```python
from build123d import *

# Parameters (mm, degrees)
ESBO_O1_R                = 2.5
RESSALTO_EXTRUS_O1_DEPTH = 1.26


with BuildPart() as part:
    # Esboço1 → Ressalto-extrusão1 (new body)
    with BuildSketch(Plane(origin=(0, 0, 0), x_dir=(1, 0, 0), z_dir=(0, 1, 0))):
        Polygon((-17.5, -9), (14.671572875, -9), (17.5, -7), (17.5, 9), (-17.5, 9), align=None)
        with Locations(Location((3.5, -1, 0), (0, 0, 270))):
            Circle(ESBO_O1_R, mode=Mode.SUBTRACT)
        with Locations(Location((-11.5, -1, 0), (0, 0, 270))):
            Circle(ESBO_O1_R, mode=Mode.SUBTRACT)
    extrude(amount=RESSALTO_EXTRUS_O1_DEPTH)


solid = part.part
```
Part model, mm, in its own coordinate system. Give positions to 0.01 mm unless a question says otherwise; leave off trailing zeros. Loops run counter-clockwise (first coordinate to the right, second up) from the corner with the lowest first, then second, coordinate; pieces in that order, holes last. Notation, with made-up numbers: M -12,68 L 27,68 A16 ccw 27,99 Z; hole C -22,39.5 d11. An arc over 180 degrees is marked long. Return JSON: item names as keys, results as strings.
1) Pull direction Z, two halves, no side cores. Call faces 1 (the face through (0, 1, -9)), 2 (the face through (-13.72, 0.62, 2.15)), 3 (the face through (16.07, 0.62, 8.01)), 4 (the face through (0, 0, 0)): released by +Z, released by -Z, zero draft, split by the parting line, or undercut.
Calculated:
{"face 1": "released by -Z", "face 2": "undercut", "face 3": "released by +Z", "face 4": "zero draft"}
2) Saw through at B-B, the plane x = -11.5. List the corners of the cut face in (y, z).
Calculated:
{"outline": "M 0,-9 L 1.26,-9 L 1.26,-1.5 L 0,-1.5 Z; M 0,3.5 L 1.26,3.5 L 1.26,9 L 0,9 Z"}
3) Flat gauge pins, fed straight in: pin 1 Ø4 at (x, z) = (-12, 0.5) entering from +Y; pin 2 Ø3 at (x, z) = (3.5, 1) entering from -Y. Where does each tip first touch, or does it go through?
Calculated:
{"pin 1": "stops at y = 1.26", "pin 2": "passes through"}
4) Saw through at C-C, the plane y = 0.8. List the corners of the cut face in (x, z).
Calculated:
{"outline": "M -17.5,-9 L 17.5,-9 L 17.5,7 L 14.67,9 L -17.5,9 Z; hole C -11.5,1 d5; hole C 3.5,1 d5"}
5) Drill centre lines: line 1 (X direction, y = 0.65, z = 1); line 2 (X direction, y = 1.15, z = 3); line 3 (Z direction, x = 1.5, y = 0.4). Where is each one in solid material? Low to high.
Calculated:
{"line 1": "x = -17.5 to -14, -9 to 1, 6 to 17.5", "line 2": "x = -17.5 to -13, -10 to 2, 5 to 17.5", "line 3": "z = -9 to -0.5, 2.5 to 9"}
6) Saw through at D-D, the plane x = 3. List the corners of the cut face in (y, z).
Calculated:
{"outline": "M 0,-9 L 1.26,-9 L 1.26,-1.45 L 0,-1.45 Z; M 0,3.45 L 1.26,3.45 L 1.26,9 L 0,9 Z"}
7) Saw through at A-A, the plane z = 1. List the corners of the cut face in (x, y), then the cut area to 3 significant figures.
Calculated:
{"outline": "M -17.5,0 L -14,0 L -14,1.26 L -17.5,1.26 Z; M -9,0 L 1,0 L 1,1.26 L -9,1.26 Z; M 6,0 L 17.5,0 L 17.5,1.26 L 6,1.26 Z", "area": "31.5 mm2"}
